The model under review builds one solid part; all positions refer to its coordinate system, in mm. Coordinates: 2 decimals unless noted, no trailing zeros. Write each loop counter-clockwise with the first axis right and the second up, starting at its lowest first coordinate (ties: lowest second). Pieces come first, ordered by that corner, then holes.
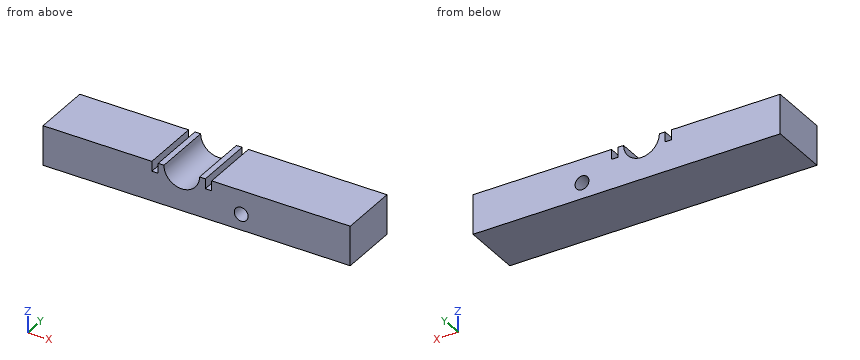
```python
from build123d import *

# Parameters (mm, degrees)
SKETCH1_W           = 155
SKETCH1_H           = 40
SKETCH1_R           = 9
BOSS_EXTRUDE1_DEPTH = 30
SKETCH3_W           = 3.175
SKETCH3_H           = 10
CUT_EXTRUDE2_DEPTH  = 31
SKETCH2_W           = 155
SKETCH2_H           = 30
CUT_EXTRUDE1_DEPTH  = 21
SKETCH4_R           = 3.5
CUT_EXTRUDE3_DEPTH  = 31


with BuildPart() as part:
    # Sketch1 → Boss-Extrude1 (new body)
    with BuildSketch(Plane(origin=(0, 0, 0), x_dir=(1, 0, 0), z_dir=(0, 1, 0))):
        with Locations((7.5, 0)):
            Rectangle(SKETCH1_W, SKETCH1_H)
        Circle(SKETCH1_R, mode=Mode.SUBTRACT)
    extrude(amount=BOSS_EXTRUDE1_DEPTH)

    # Sketch3 → Cut-Extrude2 (cut, through all)
    with BuildSketch(Plane(origin=(0, 30, 0), x_dir=(1, 0, 0), z_dir=(0, 1, 0))):
        with Locations((-13.49375, 0)):
            Rectangle(SKETCH3_W, SKETCH3_H)
        with Locations((13.49375, 0)):
            Rectangle(SKETCH3_W, SKETCH3_H)
    extrude(amount=-CUT_EXTRUDE2_DEPTH, mode=Mode.SUBTRACT)

    # Sketch2 → Cut-Extrude1 (cut, through all)
    with BuildSketch(Plane.XY):
        with Locations((7.5, 15)):
            Rectangle(SKETCH2_W, SKETCH2_H)
    extrude(amount=CUT_EXTRUDE1_DEPTH, mode=Mode.SUBTRACT)

    # Sketch4 → Cut-Extrude3 (cut, through all)
    with BuildSketch(Plane.XZ):
        with Locations((30, -12)):
            Circle(SKETCH4_R)
    extrude(amount=-CUT_EXTRUDE3_DEPTH, mode=Mode.SUBTRACT)


solid = part.part
```
Item 1: Take a section at D-D, the plane x = 0. Write out the cut boundary in (y, z).
Solved:
outline: (0, -20) - (30, -20) - (30, -9) - (0, -9) - close
Item 2: Take a section at A-A, the plane y = 4.5. Write out the cut boundary in (x, z).
Solved:
outline: (-70, -20) - (85, -20) - (85, 0) - (15.08, 0) - (15.08, -5) - (11.91, -5) - (11.91, 0) - (9, 0) arc R9 cw to (-9, 0) - (-11.91, 0) - (-11.91, -5) - (-15.08, -5) - (-15.08, 0) - (-70, 0) - close; hole circle Ø7 at (30, -12)
Item 3: Take a section at C-C, the plane x = 30. Write out the cut boundary in (y, z).
Solved:
outline: (0, -20) - (30, -20) - (30, -15.5) - (0, -15.5) - close; (0, -8.5) - (30, -8.5) - (30, 0) - (0, 0) - close
Item 4: To check wall thickness, follow line 1 along Z through (x, y) = (30, 18); line 2 along X through (y, z) = (28.5, -1); line 3 along X through (y, z) = (28.75, -2). State the ranges of each line that lie inside material, in increasing order.
Solved:
line 1: z = -20 to -15.5, -8.5 to 0
line 2: x = -70 to -15.08, -11.91 to -8.94, 8.94 to 11.91, 15.08 to 85
line 3: x = -70 to -15.08, -11.91 to -8.77, 8.77 to 11.91, 15.08 to 85
Item 5: Take a section at B-B, the plane z = -12. Write out the cut boundary in (x, y).
Solved:
outline: (-70, 0) - (26.5, 0) - (26.5, 30) - (-70, 30) - close; (33.5, 0) - (85, 0) - (85, 30) - (33.5, 30) - close
Item 6: For pin 1 (1 mm diameter, centred on x = 13, y = 22, fed in from +Z), flat-tipped, find the tip position at first contact; note if it passes through.
Solved:
pin 1: stops at z = -5
